Print and shaded views of the part. All mm, measured from the part's lowest x, y and z. A direction names the side the tool comes from. Round coordinates to 2 decimals unless told otherwise and drop trailing zeros. Loops run counter-clockwise (first coordinate to the right, second up) from the corner with the lowest first, then second, coordinate; pieces in that order, holes last. Notation, with made-up numbers: (48, 3.5) -> (101, 3.5) arc R16 cw to (101, 18.5) -> close; hole circle Ø10 at (-38.5, 85). An arc over 180 degrees is marked (long way). Answer as CSV lines item,"result".
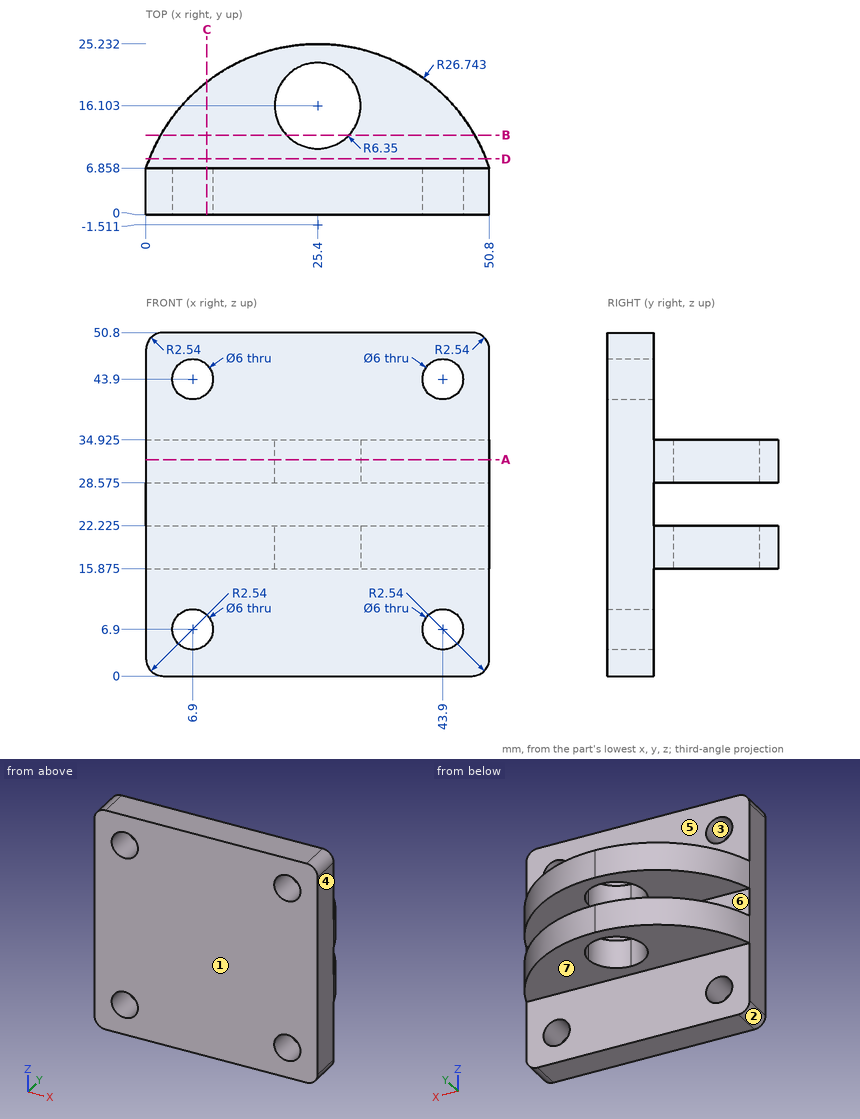
Q1. Saw through at B-B, the plane y = 11.75. Write the cut outline in (x, z) (1 decimal).
Geometry results:
outline,"(2.2, 15.9) -> (20.8, 15.9) -> (20.8, 22.2) -> (2.2, 22.2) -> close; (2.2, 28.6) -> (20.8, 28.6) -> (20.8, 34.9) -> (2.2, 34.9) -> close; (30, 15.9) -> (48.6, 15.9) -> (48.6, 22.2) -> (30, 22.2) -> close; (30, 28.6) -> (48.6, 28.6) -> (48.6, 34.9) -> (30, 34.9) -> close"
Q2. Saw through at A-A, the plane z = 32. Write the cut outline in (x, y).
Geometry results:
outline,"(0, 0) -> (50.8, 0) -> (50.8, 6.86) arc R26.74 ccw to (0, 6.86) -> close; hole circle Ø12.7 at (25.4, 16.1)"
Q3. Drill centre lines: line 1 along Z through (x, y) = (2.5, 9.5) (1 decimal); line 2 along Y through (x, z) = (25.5, 18.5); line 3 along X through (y, z) = (5.5, 6). Where is each one in solid material? Low to high.
Geometry results:
line 1,"15.9 to 22.2, 28.6 to 34.9"
line 2,"0 to 9.75, 22.45 to 25.23"
line 3,"0 to 4.04, 9.76 to 41.04, 46.76 to 50.8"
Q4. Saw through at D-D, the plane y = 8.25. Write the cut outline in (x, z) (1 decimal).
Geometry results:
outline,"(0.5, 15.9) -> (50.3, 15.9) -> (50.3, 22.2) -> (0.5, 22.2) -> close; (0.5, 28.6) -> (50.3, 28.6) -> (50.3, 34.9) -> (0.5, 34.9) -> close"
Q5. Drop flat-ended pins along their axis: P1, Ø3, axis at x = 33.5, z = 24, coming from the +Y side; P2, Ø6, axis at x = 16.5, y = 13.5, coming from the +Z side (3 decimals); P3, Ø9, axis at x = 28, y = 19, coming from the -Z side (3 decimals). Give the stop position or say it passes through.
Geometry results:
P1,"y = 6.86"
P2,"z = 34.925"
P3,"z = 15.875"
Q6. Which spindle directions (+Z, -Z, +X, -X, +Y, -Y) get a long thin tool onto all of the face, cutting with end or side? Do the marked faces 5, 6 and 7. Say none if no direction does.
Geometry results:
face 5,"+Z, +X, -X, +Y"
face 6,"+X, -X, +Y"
face 7,"-Z, +X, -X, +Y"
Q7. Two-plate mould, pull along X, no slides. Class the marked faces 1, 2, 3 and 4: pulls with the +X half, pulls with the -X half, needs draft (parallel to the pull), parting line crosses it, or undercut.
Geometry results:
face 1,"needs draft"
face 2,"pulls with the -X half"
face 3,"undercut"
face 4,"pulls with the +X half"
Q8. Saw through at C-C, the plane x = 9. Write the cut outline in (y, z) (1 decimal).
Geometry results:
outline,"(0, 0) -> (6.9, 0) -> (6.9, 4.8) -> (0, 4.8) -> close; (0, 9) -> (6.9, 9) -> (6.9, 15.9) -> (19.6, 15.9) -> (19.6, 22.2) -> (6.9, 22.2) -> (6.9, 28.6) -> (19.6, 28.6) -> (19.6, 34.9) -> (6.9, 34.9) -> (6.9, 41.8) -> (0, 41.8) -> close; (0, 46) -> (6.9, 46) -> (6.9, 50.8) -> (0, 50.8) -> close"
